```python
from build123d import *

# Parameters (mm, degrees)
F1_DEPTH = 508
F3_W     = 91.848578011
F3_H     = 482.6
F4_DEPTH = 50.8
F2_R     = 3.175
F5_DEPTH = 12.7
F6_DEPTH = 3.175
F7_DEPTH = 3.175


with BuildPart() as f1:
    # F0 (on Front) → F1 (new body)
    with BuildSketch(Plane.XZ):
        Polygon((31.3197647862, -27.9812486264), (35.8098928468, -32.4713766869), (170.1866526071, 101.9053830735), (120.1831479018, 136.9182140051), (16.6587981808, 81.8733408519), (39.4792327577, -19.8217806548), align=None)
    extrude(amount=F1_DEPTH)

    # F3 (on face) → F4 (cut)
    with BuildSketch(Plane(origin=(-30.2663796495, 0, 56.9227812171), x_dir=(0.8829475929, 0, 0.4694715628), z_dir=(-0.4694715628, 0, 0.8829475929))):
        with Locations((111.7703400394, -254)):
            Rectangle(F3_W, F3_H)
    extrude(amount=-F4_DEPTH, mode=Mode.SUBTRACT)

    # F2 (on face) → F5 (cut)
    with BuildSketch(Plane(origin=(34.1406347668, 0, -34.1406347668), x_dir=(0.7071067812, 0, 0.7071067812), z_dir=(0.7071067812, 0, -0.7071067812))):
        with Locations((38.4032874157, 486.6894)):
            Circle(F2_R)
    extrude(amount=-F5_DEPTH, mode=Mode.SUBTRACT)

    # F6 (add): a face of the model
    f6_faces = [f1.faces().sort_by_distance(p)[0] for p in [
        (82.8731770795, -508, 66.5046152241),
    ]]
    extrude(f6_faces, amount=F6_DEPTH)

    # F7 (add): a face of the model
    f7_faces = [f1.faces().sort_by_distance(p)[0] for p in [
        (82.8731770795, 0, 66.5046152241),
    ]]
    extrude(f7_faces, amount=F7_DEPTH)


solid = f1.part
```
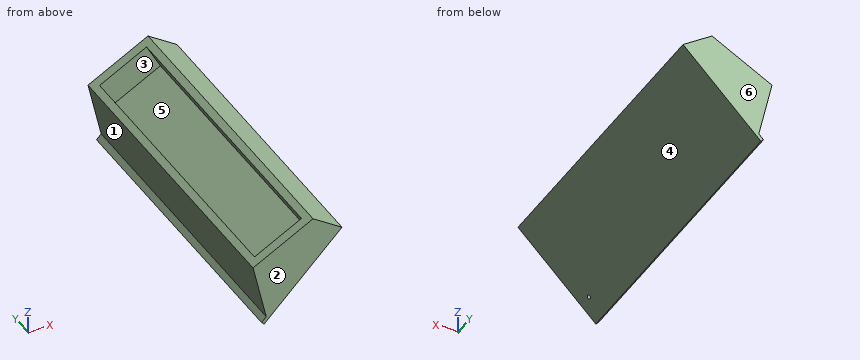
Could you check a few things on this model? Use its own coordinates, in mm. Face numbers are marked on the shaded views. A direction names the side the tool comes from. Give positions to 0.01 mm unless a question says otherwise; leave off trailing zeros. Write each loop counter-clockwise with the first axis right and the second up, starting at its lowest first coordinate (ties: lowest second). Pieces come first, ordered by that corner, then holes. Notation, with made-up numbers: (-30.75, 24) - (-16.75, 24) arc R18 ccw to (-16.75, 41) - close; hole circle Ø6 at (1.5, -38.75). An arc over 180 degrees is marked (long way). One line per item, written item: value. Start each with the question number.
Item 1: If we mould it in two halves opening along Y, with no side actions, what happens to the marked faces 4, 5 and 6? For each: +Y half, -Y half, draft (parallel to the pull), parting line (faces both ways), or undercut.
Item 2: Imagine slicing it at B-B, the plane y = -307. List the corners of the cut face in (x, z) for me, and give its area (3 significant figures).
Item 3: Imagine slicing it at C-C, the plane x = 77.5. List the corners of the cut face in (y, z) for me (3 decimals).
Item 4: Which directions (+Z, -Z, +X, -X, +Y, -Y) give clear straight access to the entire face, cutting with the end or side of a thin tool? Please do the marked faces 1, 2 and 3.
Item 5: I'm going to push flat-ended pins straight in: pin 1 (1.5 mm diameter, centred on x = 152, y = -90.5, fed in from +Z); pin 2 (6 mm diameter, centred on x = 47.5, y = -177.5, fed in from +Z); pin 3 (4 mm diameter, centred on x = 151.5, y = -73, fed in from -Z). Where does each tip first touch, or does it pass through?
Item 6: Imagine slicing it at D-D, the plane z = 65.5. List the corners of the cut face in (x, y) for me (3 decimals).
Item 7: Imagine slicing it at A-A, the plane z = 111. List the corners of the cut face in (x, y) for me (3 decimals).
Item 8: Please list where these lines run through material, in increasing order: line 1 (Y direction, x = 48.5, z = 58) (3 decimals); line 2 (Z direction, x = 68, y = -184); line 3 (X direction, y = -300.5, z = 49.5). Write a range as from..to.
Geometry says:
1. face 4: draft
1. face 5: undercut
1. face 6: +Y half
2. outline: (16.66, 81.87) - (39.48, -19.82) - (31.32, -27.98) - (35.81, -32.47) - (170.19, 101.91) - (120.18, 136.92) - (108.97, 130.96) - (132.82, 86.1) - (51.72, 42.98) - (27.87, 87.84) - close
2. area: 7,200 mm^2
3. outline: (-511.175, 9.219) - (3.175, 9.219) - (3.175, 114.223) - (-12.7, 114.223) - (-12.7, 56.689) - (-495.3, 56.689) - (-495.3, 114.223) - (-511.175, 114.223) - close
4. face 1: -X, +Y, -Y
4. face 2: +Z, -Z, +X, -X, -Y
4. face 3: none
5. pin 1: z = 115.16
5. pin 2: z = 56.56
5. pin 3: z = 81.22
6. outline: (20.333, -511.175) - (133.781, -511.175) - (133.781, 3.175) - (20.333, 3.175) - close; hole (39.748, -495.3) - (94.072, -495.3) - (94.072, -12.7) - (39.748, -12.7) - close
7. outline: (71.438, -511.175) - (157.198, -511.175) - (157.198, 3.175) - (71.438, 3.175) - (71.438, -12.7) - (119.58, -12.7) - (119.58, -495.3) - (71.438, -495.3) - close
8. line 1: -511.175..-495.3, -12.7..3.175
8. line 2: -0.28..51.64
8. line 3: 23.92..48.26, 63.98..117.78
